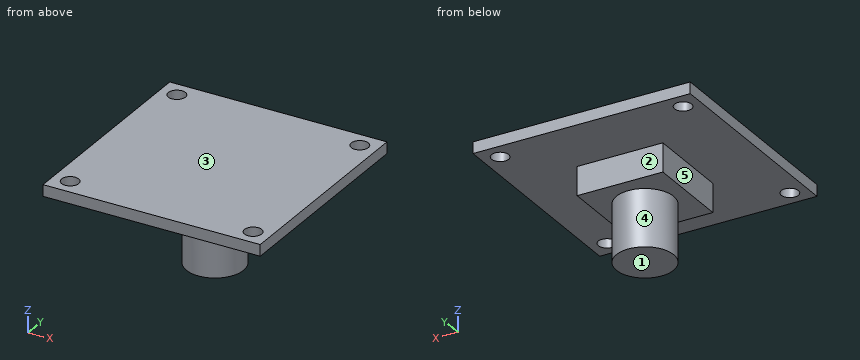
from build123d import *

# Parameters (mm, degrees)
F0_W      = 38
F0_H      = 38
F0_R      = 1.5
F1_DEPTH  = 2
F2_W      = 15
F2_H      = 15
F2_R      = 5
F3_DEPTH  = 5
F3_FACE_R = 5
F4_DEPTH  = 15


with BuildPart() as f1:
    # F0 (on Top) → F1 (new body)
    with BuildSketch(Plane.XY):
        Rectangle(F0_W, F0_H)
        with Locations((-16, -16)):
            Circle(F0_R, mode=Mode.SUBTRACT)
        with Locations((16, -16)):
            Circle(F0_R, mode=Mode.SUBTRACT)
        with Locations((-16, 16)):
            Circle(F0_R, mode=Mode.SUBTRACT)
        with Locations((16, 16)):
            Circle(F0_R, mode=Mode.SUBTRACT)
    extrude(amount=F1_DEPTH)

    # F2 (on face) → F3 (join)
    with BuildSketch(Plane(origin=(0, 0, 0), x_dir=(1, 0, 0), z_dir=(0, 0, -1))):
        Rectangle(F2_W, F2_H)
        Circle(F2_R, mode=Mode.SUBTRACT)
    extrude(amount=F3_DEPTH)

    # F3_face (on face) → F4 (join)
    with BuildSketch(Plane(origin=(0, 0, 0), x_dir=(1, 0, 0), z_dir=(0, 0, -1))):
        Circle(F3_FACE_R)
    extrude(amount=F4_DEPTH)


solid = f1.part
Build history of the part. All positions in model axes, mm. Face numbers are marked on the shaded views. A direction names the side the tool comes from. Coordinates: 2 decimals unless noted, no trailing zeros. Write each loop counter-clockwise with the first axis right and the second up, starting at its lowest first coordinate (ties: lowest second). Pieces come first, ordered by that corner, then holes. Notation, with made-up numbers: (47.25, 9.25) -> (76.25, 9.25) arc R24 cw to (76.25, 41.25) -> close; hole circle Ø11 at (45, 88.25). An arc over 180 degrees is marked (long way). Use CSV: the item, a comma, the result in double quotes. Start each with the question number.
Q1. Cut at A-A, the plane x = 16. List the corners of the cut face in (y, z).
Q2. Drill centre lines: probe 1 along Y at (x, z) = (-16, 1.65); probe 2 along Z at (x, y) = (17, 14.5); probe 3 along X at (y, z) = (4.5, -4.25). Where is each one in solid material? Low to high.
Q3. Cut at C-C, the plane y = 0. List the corners of the cut face in (x, z), then the cut area to 3 significant figures.
Q4. Flat gauge pins, fed straight in: pin 1 Ø2.5 at (x, y) = (16, -16) entering from +Z; pin 2 Ø2 at (x, y) = (0.5, 6.5) entering from -Z; pin 3 Ø4 at (x, y) = (16, 16) entering from -Z; pin 4 Ø10 at (x, z) = (7, -12) entering from -Y. Where does each tip first touch, or does it go through?
Q5. 3-axis set-ups, long thin cutter, end or side, ignore diameter. For the marked faces 1, 2, 3, 4 and 5: which of +Z, -Z, +X, -X, +Y, -Y reach the whole face in a straight line?
Checked values:
1,outline,"(-19, 0) -> (-17.5, 0) -> (-17.5, 2) -> (-19, 2) -> close; (-14.5, 0) -> (14.5, 0) -> (14.5, 2) -> (-14.5, 2) -> close; (17.5, 0) -> (19, 0) -> (19, 2) -> (17.5, 2) -> close"
2,probe 1,"y = -19 to -17.5, -14.5 to 14.5, 17.5 to 19"
2,probe 2,"z = 0 to 2"
2,probe 3,"x = -7.5 to 7.5"
3,outline,"(-19, 0) -> (-7.5, 0) -> (-7.5, -5) -> (-5, -5) -> (-5, -15) -> (5, -15) -> (5, -5) -> (7.5, -5) -> (7.5, 0) -> (19, 0) -> (19, 2) -> (-19, 2) -> close"
3,area,"251 mm²"
4,pin 1,"passes through"
4,pin 2,"stops at z = -5"
4,pin 3,"stops at z = 0"
4,pin 4,"stops at y = -4.58"
5,face 1,"-Z, +X, -X, +Y, -Y"
5,face 2,"-Z, +X, -X, +Y"
5,face 3,"+Z, +X, -X, +Y, -Y"
5,face 4,"-Z"
5,face 5,"-Z, -X, +Y, -Y"
